Part model, mm, in its own coordinate system. Round coordinates to 2 decimals unless told otherwise and drop trailing zeros. Loops run counter-clockwise (first coordinate to the right, second up) from the corner with the lowest first, then second, coordinate; pieces in that order, holes last.
(1) Cut at B-B on z = 375. List the corners of the cut face in (x, y).
(2) Probe probe 1 along X at (y, z) = (6, 185); probe 2 along X at (y, z) = (1.85, 360); probe 3 along X at (y, z) = (6, 177.5). List the from-to ranges inside material, lowest first.
(3) Cut at A-A on y = 2. Count the separate pieces of the cut face and the enclosed holes in it, then the cut area to 3 significant figures.
(4) Flat gauge pin, fed straight in: pin 1 (5.5 mm diameter, centred on x = 6, z = 410, fed in from +Y). Where does the tip first touch, or does it go through?
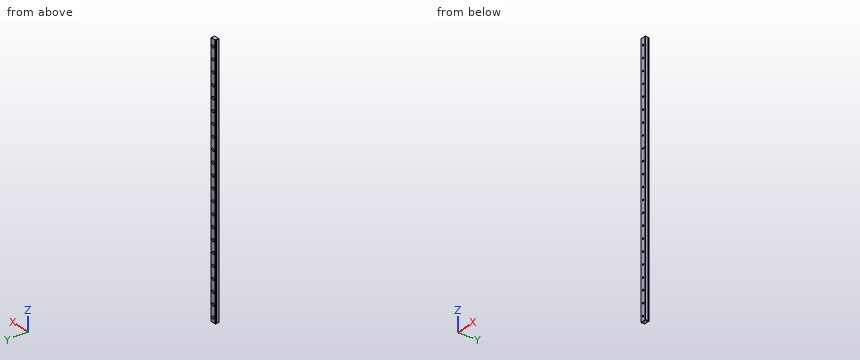
from build123d import *

# Parameters (mm, degrees)
BOSS_EXTRUDE1_DEPTH         = 550
CHAMFER1_SIZE               = 0.3
HOLE_WIZARD_M51_D           = 3.5
HOLE_WIZARD_M51_CBORE_D     = 6
HOLE_WIZARD_M51_CBORE_DEPTH = 4.5
LPATTERN1_COUNT             = 22
LPATTERN1_PITCH             = 25


with BuildPart() as part:
    # Sketch1 → Boss-Extrude1 (new body)
    with BuildSketch(Plane.XY):
        with BuildLine():
            Line((0, 8), (12, 8))
            Line((12, 8), (12, 6.75))
            Line((12, 6.75), (12, 6.559016994))
            ThreePointArc((12, 6.559016994), (11.706107374, 6.475528258), (11.5, 6.25))
            Line((11.5, 6.25), (11, 6.25))
            Line((11, 6.25), (11, 5.75))
            Line((11, 5.75), (11.5, 5.75))
            ThreePointArc((11.5, 5.75), (11.706107374, 5.524471742), (12, 5.440983006))
            Line((12, 5.440983006), (12, 5.25))
            Line((12, 5.25), (12, 0))
            Line((12, 0), (0, 0))
            Line((0, 0), (0, 5.25))
            Line((0, 5.25), (0, 5.440983006))
            ThreePointArc((0, 5.440983006), (0.293892626, 5.524471742), (0.5, 5.75))
            Line((0.5, 5.75), (1, 5.75))
            Line((1, 5.75), (1, 6.25))
            Line((1, 6.25), (0.5, 6.25))
            ThreePointArc((0.5, 6.25), (0.293892626, 6.475528258), (0, 6.559016994))
            Line((0, 6.559016994), (0, 6.75))
            Line((0, 6.75), (0, 8))
        make_face()
    extrude(amount=BOSS_EXTRUDE1_DEPTH)

    # Chamfer1
    chamfer1_edges = [part.edges().sort_by_distance(p)[0] for p in [
        (12, 2.720491503, 550),
        (11.706107374, 5.524471742, 550),
        (0, 2.720491503, 0),
        (0.293892626, 5.524471742, 0),
        (0.75, 5.75, 0),
        (1, 6, 0),
        (0.75, 6.25, 0),
        (11.25, 5.75, 550),
        (0.293892626, 6.475528258, 0),
        (0, 7.279508497, 0),
        (6, 8, 0),
        (12, 7.279508497, 0),
        (11.706107374, 6.475528258, 0),
        (11, 6, 550),
        (11.25, 6.25, 0),
        (11, 6, 0),
        (11.25, 5.75, 0),
        (11.706107374, 5.524471742, 0),
        (12, 2.720491503, 0),
        (6, 0, 0),
        (11.25, 6.25, 550),
        (11.706107374, 6.475528258, 550),
        (12, 7.279508497, 550),
        (0, 8, 275),
        (12, 8, 275),
        (12, 0, 275),
        (0, 0, 275),
        (6, 8, 550),
        (0, 2.720491503, 550),
        (0, 7.279508497, 550),
        (0.293892626, 6.475528258, 550),
        (0.75, 6.25, 550),
        (1, 6, 550),
        (0.75, 5.75, 550),
        (0.293892626, 5.524471742, 550),
        (6, 0, 550),
    ]]
    chamfer(chamfer1_edges, length=CHAMFER1_SIZE)

    # Цековка для  болта с шестигранной головкой M51 (through all)
    with Locations(Plane(origin=(6, 8, 10), x_dir=(0, 0, 1), z_dir=(0, 1, 0))):
        with Locations((0, 0)):
            hole_wizard_m51 = CounterBoreHole(HOLE_WIZARD_M51_D / 2, HOLE_WIZARD_M51_CBORE_D / 2, HOLE_WIZARD_M51_CBORE_DEPTH)

    # LPattern1: Цековка для  болта с шестигранной головкой M51 ×22
    with Locations(*[(0, 0, i * LPATTERN1_PITCH) for i in range(1, LPATTERN1_COUNT)]):
        add(hole_wizard_m51, mode=Mode.SUBTRACT)


solid = part.part
Final values:
1. outline: (0, 0.3) - (0.3, 0) - (11.7, 0) - (12, 0.3) - (12, 5.44) arc R0.56 cw to (11.5, 5.75) - (11, 5.75) - (11, 6.25) - (11.5, 6.25) arc R0.56 cw to (12, 6.56) - (12, 7.7) - (11.7, 8) - (0.3, 8) - (0, 7.7) - (0, 6.56) arc R0.56 cw to (0.5, 6.25) - (1, 6.25) - (1, 5.75) - (0.5, 5.75) arc R0.56 cw to (0, 5.44) - close
2. probe 1: x = 1 to 3, 9 to 11
2. probe 2: x = 0 to 4.25, 7.75 to 12
2. probe 3: x = 1 to 11
3. separate pieces: 1
3. enclosed holes: 22
3. area: 6,390 mm2
4. pin 1: stops at y = 3.5
